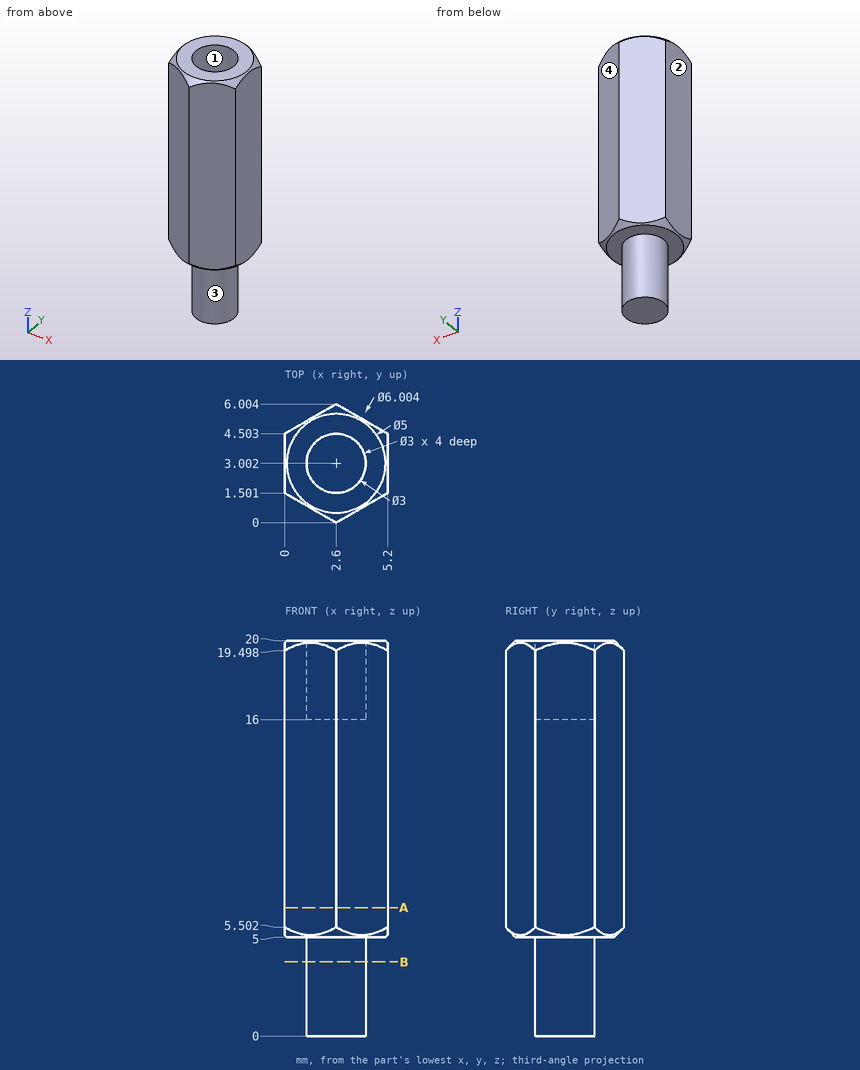
Answer from the drawing. Dimensions are ordinates in mm from the lowest x, y and z of the part. Coordinates: 2 decimals unless noted, no trailing zeros. Write each loop counter-clockwise with the first axis right and the second up, starting at its lowest first coordinate (ties: lowest second). Pieces come first, ordered by that corner, then holes. Notation, with made-up numbers: (-14, 18.5) - (-9, 18.5) arc R21 ccw to (-9, 52.5) - close; hole circle Ø10 at (22, 21). An arc over 180 degrees is marked (long way). Return JSON: item names as keys, results as strings.
1. The part is cut by section A-A on z = 6.5. Determine the outline of the cut face in (x, y) (1 decimal).
Final values:
{"outline": "(0, 1.5) - (2.6, 0) - (5.2, 1.5) - (5.2, 4.5) - (2.6, 6) - (0, 4.5) - close"}
2. The part is cut by section B-B on z = 3.75. Determine the outline of the cut face in (x, y).
Final values:
{"outline": "circle Ø3 at (2.6, 3)"}
3. Consider line 1 along Z through (x, y) = (0.45, 2.25); line 2 along Y through (x, z) = (3.75, 18.5) (1 decimal); line 3 along Y through (x, z) = (3.65, 10) (1 decimal). Determine where each line is inside the solid, lowest interval first.
Final values:
{"line 1": "5 to 20", "line 2": "0.7 to 2, 4 to 5.3", "line 3": "0.6 to 5.4"}
4. For a pull along Y with two mould halves and no side action, classify the marked faces 1, 2, 3 and 4 as +Y half, -Y half, draft (parallel to the pull), parting line (faces both ways), or undercut.
Final values:
{"face 1": "undercut", "face 2": "draft", "face 3": "parting line", "face 4": "+Y half"}
